Could you check a few things on this model? Use its own coordinates, in mm. A direction names the side the tool comes from. Coordinates: 2 decimals unless noted, no trailing zeros. Loops run counter-clockwise (first coordinate to the right, second up) from the corner with the lowest first, then second, coordinate; pieces in that order, holes last. Notation, with made-up numbers: (22.5, 44) - (41.5, 44) arc R19 cw to (41.5, 66) - close; hole circle Ø2 at (-23, -1.75). An arc over 180 degrees is marked (long way). Put each result on its own line as item: value. Start each with the question number.
Autodesk Inventor part; units mm, degrees
ref_plane "YZ Plane" through (0, 0, 0) normal (1, 0, 0) x (0, 1, 0)
ref_plane "XZ Plane" through (0, 0, 0) normal (0, 1, 0) x (-1, 0, 0)
ref_plane "XY Plane" through (0, 0, 0) normal (0, 0, 1) x (1, 0, 0)
sketch "Sketch1" plane through (0, 0, 0) normal (0, 1, 0) x (-1, 0, 0)
  line L0 (-6, -11.5) -> (6, -11.5)
  line L1 (6, -11.5) -> (6, 11.5)
  line L2 (6, 11.5) -> (-6, 11.5)
  line L3 (-6, 11.5) -> (-6, -11.5)
  line L4 (-6, -11.5) -> (6, 11.5) construction
  line L5 (6, -11.5) -> (-6, 11.5) construction
  point P0 (0, 0)
  dimension "d0" = 12
  dimension "d1" = 23
extrude "Extrusion1" add sketch "Sketch1" along normal blind 23.5
sketch "Sketch2" plane through (-6, 0, -11.5) normal (-1, 0, 0) x (0, 0, 1)
  line L0 (0, 23.5) -> (23, 23.5)
  line L1 (0, 18.5) -> (23, 18.5)
  line L2 (0, 18.5) -> (0, 16.523)
  line L3 (0, 16.523) -> (23, 16.523)
  line L4 (23, 16.523) -> (23, 18.5)
  point P0 (11.5, 0)
  dimension "d7" = 5
extrude "Extrusion2" add sketch "Sketch2" along normal blind 5
sketch "Sketch3" plane through (6, 0, 11.5) normal (1, 0, 0) x (0, 0, -1)
  line L0 (0, 16.523) -> (0, 18.5)
  line L1 (0, 18.5) -> (23, 18.5)
  line L2 (23, 18.5) -> (23, 16.523)
  line L3 (23, 16.523) -> (0, 16.523)
  point P0 (11.5, 0)
extrude "Extrusion3" add sketch "Sketch3" along normal blind 5
sketch "Sketch4" plane through (0, 23.5, 0) normal (0, 1, 0) x (1, 0, 0)
  circle A0 centre (0, 5.5) radius 6
  line L0 (6, 11.5) -> (-6, 11.5)
  point P0 (0, 0)
  dimension "d12" = 12
  dimension "d13" = 6
extrude "Extrusion4" add sketch "Sketch4" along normal blind 4
sketch "Sketch6" plane through (0, 23.5, 0) normal (0, 1, 0) x (1, 0, 0)
  circle A0 centre (0, -2) radius 3
  point P0 (0, 0)
  dimension "d17" = 6
extrude "Extrusion5" add sketch "Sketch6" along normal up to surface (4 mm away)
sketch "Sketch7" plane through (-6, 0, 11.5) normal (0, 0, 1) x (1, 0, 0)
  line L0 (12, 18.5) -> (17, 18.5)
  line L1 (0, 18.5) -> (-5, 18.5)
  line L2 (0, 16.523) -> (-5, 16.523)
  line L3 (12, 16.523) -> (17, 16.523)
  line L4 (0, 18.5) -> (0, 16.523)
  line L5 (0, 16.523) -> (12, 16.523)
  line L6 (12, 16.523) -> (12, 18.5)
  line L7 (0, 18.5) -> (12, 18.5)
  point P0 (6, 0)
extrude "Extrusion6" add sketch "Sketch7" along normal blind 5
sketch "Sketch8" plane through (6, 0, -11.5) normal (0, 0, -1) x (-1, 0, 0)
  line L0 (0, 18.5) -> (12, 18.5)
  line L1 (12, 18.5) -> (12, 16.523)
  line L2 (12, 16.523) -> (0, 16.523)
  line L3 (0, 16.523) -> (0, 18.5)
  point P0 (6, 0)
extrude "Extrusion7" add sketch "Sketch8" along normal blind 5
sketch "Sketch9" plane through (11, 0, 11.5) normal (1, 0, 0) x (0, 0, -1)
  line L0 (23, 16.523) -> (23, 18.5)
  line L1 (23, 18.5) -> (0, 18.5)
  line L2 (0, 18.5) -> (0, 16.523)
  line L3 (0, 16.523) -> (23, 16.523)
  point P0 (11.5, 0)
extrude "Extrusion8" cut sketch "Sketch9" against normal up to surface (5 mm away)
sketch "Sketch10" plane through (-11, 0, -11.5) normal (-1, 0, 0) x (0, 0, 1)
  line L0 (23, 16.523) -> (23, 18.5)
  line L1 (23, 18.5) -> (0, 18.5)
  line L2 (0, 18.5) -> (0, 16.523)
  line L3 (0, 16.523) -> (23, 16.523)
  point P0 (11.5, 0)
extrude "Extrusion9" cut sketch "Sketch10" against normal up to surface (5 mm away)
sketch "Sketch11" plane through (0, 27.5, 0) normal (0, 1, 0) x (1, 0, 0)
  circle A0 centre (0, 5.5352) radius 3.5
  point P0 (0, 0)
  dimension "d28" = 7
extrude "Extrusion10" add sketch "Sketch11" along normal blind 5
sketch "Sketch14" plane through (0, 32.5, -5.5352) normal (0, 1, 0) x (1, 0, 0)
  line L0 (-2, -3) -> (2, -3)
  line L1 (2, -3) -> (2, -15.5)
  line L2 (2, -15.5) -> (-2, -15.5)
  line L3 (-2, -15.5) -> (-2, -3)
  line L4 (-2, 3) -> (2, 3)
  line L5 (2, 3) -> (2, 15.5)
  line L6 (2, 15.5) -> (-2, 15.5)
  line L7 (-2, 15.5) -> (-2, 3)
  point P0 (0, -5.5352)
  dimension "d39" = 12.5
  dimension "d40" = 12.5
extrude "Extrusion13" add sketch "Sketch14" against normal blind 1.5
properties part number "Servo" material "S355J2+N"
(1) If we mould it in two halves opening along Z, with no side actions, what happens to faces 1 (the flat face through (0, 18, -16.5)), 2 (the flat face through (0, 32, 9.965)), 3 (the cylindrical face through (0, 25, 5)), 4 (the flat face through (-2, 32, 4))? For each: pulls with the +Z half, pulls with the -Z half, needs draft (parallel to the pull), parting line crosses it, or undercut.
(2) I need wall thicknesses on L1, parallel to Y at x = 1.75, z = -0.5; L2, parallel to Y at x = -2, z = 12.5; L3, parallel to Z at x = -2.5, y = 12. Which ranges of each line are inside material? Lowest first, please. Write a range as [from, to].
(3) I want a section at C-C on z = 7.5. List the corners of the cut face in (x, y) for me.
(4) I want a section at A-A on z = 2. List the corners of the cut face in (x, y) for me, and give its area (3 significant figures).
(5) I want a section at D-D on z = -7. List the corners of the cut face in (x, y) for me.
(6) For pin 1 Ø1.6 at (y, z) = (32, 6) entering from +X; pin 2 Ø2.5 at (x, y) = (-1.5, 20) entering from +Z; pin 3 Ø3.5 at (x, y) = (2, 8.5) entering from -Z, each with a flat end and sliding along its axis, tell me the tip position at first contact or that it passes through.
(7) Which directions (+Z, -Z, +X, -X, +Y, -Y) give clear straight access to the entire face, cutting with the end or side of a thin tool? Please do faces 5 (the flat face through (0, 18.5, -14)), 6 (the flat face through (0, 16.523, 14)), 7 (the flat face through (0, 16.523, -14)), 8 (the flat face through (0, 21, 11.5)), 9 (the flat face through (2, 32, 4)).
(8) I want a section at B-B on x = 4.75. List the corners of the cut face in (y, z) for me, and give its area (3 significant figures).
Answer sheet:
1. face 1: pulls with the -Z half
1. face 2: pulls with the +Z half
1. face 3: undercut
1. face 4: needs draft
2. L1: y = [0, 27.5], [31, 32.5]
2. L2: y = [16.52, 18.5]
2. L3: z = [-11.5, 11.5]
3. outline: (-6, 0) - (6, 0) - (6, 23.5) - (-6, 23.5) - close; (-2, 31) - (2, 31) - (2, 32.5) - (-2, 32.5) - close
4. outline: (-6, 0) - (6, 0) - (6, 23.5) - (3, 23.5) - (3, 27.5) - (-3, 27.5) - (-3, 23.5) - (-6, 23.5) - close; (-2, 31) - (2, 31) - (2, 32.5) - (-2, 32.5) - close
4. area: 312 mm^2
5. outline: (-6, 0) - (6, 0) - (6, 23.5) - (5.81, 23.5) - (5.81, 27.5) - (3.18, 27.5) - (3.18, 32.5) - (-3.18, 32.5) - (-3.18, 27.5) - (-5.81, 27.5) - (-5.81, 23.5) - (-6, 23.5) - close
6. pin 1: stops at x = 2
6. pin 2: stops at z = 11.5
6. pin 3: stops at z = -11.5
7. face 5: -Z, +X, -X
7. face 6: +Z, +X, -X, -Y
7. face 7: -Z, +X, -X, -Y
7. face 8: +Z, +X, -X, +Y
7. face 9: +Z, +X, +Y
8. outline: (0, -11.5) - (16.52, -11.5) - (16.52, -16.5) - (18.5, -16.5) - (18.5, -11.5) - (23.5, -11.5) - (23.5, -9.17) - (27.5, -9.17) - (27.5, -1.83) - (23.5, -1.83) - (23.5, 11.5) - (18.5, 11.5) - (18.5, 16.5) - (16.52, 16.5) - (16.52, 11.5) - (0, 11.5) - close
8. area: 590 mm^2
